```python
from build123d import *

# Parameters (mm, degrees)
SKETCH1_W          = 1.5875
SKETCH1_H          = 76.9
CUT_EXTRUDE3_START = -9.525
CUT_EXTRUDE3_DEPTH = 9.525
CUT_EXTRUDE4_DEPTH = 9.525


# Read off the part's stored shape, not the designer's step: Tap Drill for #10-32 Tap1
with BuildPart() as part:
    # Sketch1 → Revolve1 (revolve)
    with BuildSketch(Plane.XY, mode=Mode.PRIVATE) as revolve1_sk:
        with Locations((-3.96875, 0)):
            Rectangle(SKETCH1_W, SKETCH1_H)
        Polygon((0, -57.5), (-4.7625, -57.5), (-4.7625, -38.45), (-3.175, -38.45), (-3.175, 38.45), (-4.7625, 38.45), (-4.7625, 57.5), (0, 57.5), align=None)
    revolve(revolve1_sk.sketch.rotate(Axis((0, -57.5, 0), (0, 1, 0)), 180), axis=Axis((0, -57.5, 0), (0, 1, 0)))

    # Sketch2 → Cut-Extrude3 (cut)
    with BuildSketch(Plane.XZ.offset(57.5).offset(CUT_EXTRUDE3_START)):
        with BuildLine():
            Line((-3.96875, -2.632570927), (-3.96875, 2.632570927))
            ThreePointArc((-3.96875, 2.632570927), (-4.7625, 0), (-3.96875, -2.632570927))
        make_face()
        with BuildLine():
            Line((3.96875, -2.632570927), (3.96875, 2.632570927))
            ThreePointArc((3.96875, 2.632570927), (4.7625, 0), (3.96875, -2.632570927))
        make_face()
    extrude(amount=CUT_EXTRUDE3_DEPTH, mode=Mode.SUBTRACT)

    # Sketch5 → Cut-Extrude4 (cut)
    with BuildSketch(Plane(origin=(0, 57.5, 0), x_dir=(1, 0, 0), z_dir=(0, 1, 0))):
        with BuildLine():
            Line((-3.96875, -2.632570927), (-3.96875, 2.632570927))
            ThreePointArc((-3.96875, 2.632570927), (-4.7625, 0), (-3.96875, -2.632570927))
        make_face()
        with BuildLine():
            Line((3.96875, -2.632570927), (3.96875, 2.632570927))
            ThreePointArc((3.96875, 2.632570927), (4.7625, 0), (3.96875, -2.632570927))
        make_face()
    extrude(amount=-CUT_EXTRUDE4_DEPTH, mode=Mode.SUBTRACT)

    # Tap Drill for #10-32 Tap1 outline → Tap Drill for #10-32 Tap1 (revolve, cut)
    with BuildSketch(Plane.XY):
        Polygon((0, 57.5), (0, 40.284682152), (2.0193, 41.498), (2.0193, 57.5), align=None)
        Polygon((2.0193, -41.498), (0, -40.284682152), (0, -57.5), (2.0193, -57.5), align=None)
    revolve(axis=Axis((0, 0, 0), (0, 1, 0)), mode=Mode.SUBTRACT)


solid = part.part
```
Geometry check sheet. Reference: the model listing, model coordinates, mm. A direction names the side the tool comes from. Give positions to 0.01 mm unless a question says otherwise; leave off trailing zeros. Loops run counter-clockwise (first coordinate to the right, second up) from the corner with the lowest first, then second, coordinate; pieces in that order, holes last. Notation, with made-up numbers: (-22, 30.5) - (-18, 30.5) arc R27 cw to (-18, 46.5) - close; hole circle Ø7 at (-14, 37). An arc over 180 degrees is marked (long way). Use CSV: the item, a comma, the result in double quotes. Start each with the question number.
Q1. Section check A-A, the plane y = 5. Record the cut outline in (x, z) (1 decimal), and give its area (3 significant figures).
Q2. Access from +Z, -Z, +X, -X, +Y, -Y to the whole of each face (thin tool, end or side, straight path). Record for faces 4 (the face through (3.969, -53, 0)), 5 (the face through (1.926, -49.387, -0.607)), 6 (the face through (3.969, 53, 0)).
Q3. Go/stop test with flat-tipped pins: pin 1 Ø4 at (y, z) = (-53.5, 0.5) entering from +X; pin 2 Ø4 at (y, z) = (54, 1) entering from -X; pin 3 Ø2.5 at (x, z) = (0, 0) entering from -Y. Record where each tip stops, or that it passes through.
Q4. Release check for a two-part mould opening along Z. For faces 1 (the face through (-3.969, 53, 0)), 2 (the face through (-4.758, -0.805, -0.209)), 3 (the face through (-0.076, 40.495, 0.342)) record: +Z half, -Z half, draft (parallel to the pull), parting line (faces both ways), or undercut.
Q5. Scan lines: probe 1 along X at (y, z) = (-53.5, 0); probe 2 along Z at (x, y) = (-0.25, -23); probe 3 along X at (y, z) = (49, 1.25). Record each from-to range of solid material in increasing order. Write a range as from..to.
Findings below:
1,outline,"circle Ø9.5 at (0, 0)"
1,area,"71.3 mm^2"
2,face 4,"+Z, -Z, +X, -Y"
2,face 5,"-Y"
2,face 6,"+Z, -Z, +X, +Y"
3,pin 1,"stops at x = 3.97"
3,pin 2,"stops at x = -3.97"
3,pin 3,"stops at y = -41.04"
4,face 1,"draft"
4,face 2,"parting line"
4,face 3,"undercut"
5,probe 1,"x = -3.97..-2.02, 2.02..3.97"
5,probe 2,"z = -4.76..4.76"
5,probe 3,"x = -3.97..-1.59, 1.59..3.97"
